Source: CAD feature listing. Evaluate the final solid. Frame: model axes, mm. A direction names the side the tool comes from. Give positions to 0.01 mm unless a question says otherwise; leave off trailing zeros. Loops run counter-clockwise (first coordinate to the right, second up) from the corner with the lowest first, then second, coordinate; pieces in that order, holes last. Notation, with made-up numbers: M 46.25,28 L 91.25,28 A26 cw 91.25,43 Z; hole C 47,10.5 d1. An arc over 180 degrees is marked long. Answer in a Markdown table with one row per item.
Autodesk Inventor part; units mm, degrees
ref_plane "YZ Plane" through (0, 0, 0) normal (1, 0, 0) x (0, 1, 0)
ref_plane "XZ Plane" through (0, 0, 0) normal (0, 1, 0) x (-1, 0, 0)
ref_plane "XY Plane" through (0, 0, 0) normal (0, 0, 1) x (1, 0, 0)
sketch "Sketch1" plane through (0, 0, 0) normal (0, 1, 0) x (-1, 0, 0)
  line L0 (0, 0) -> (19, 0) construction
  line L1 (19, -5) -> (19, -15.5)
  line L2 (19, 0) -> (16, 0) construction
  line L3 (16, 0) -> (16, -5)
  line L4 (16, -5) -> (19, -5)
  circle A0 centre (0, 0) radius 14.5
  line L5 (19, -15.5) -> (0, -15.5)
  line L6 (0, 0) -> (0, 19.3776) construction
  line L7 (19, 5) -> (19, 15.5)
  line L8 (16, 0) -> (16, 5)
  line L9 (16, 5) -> (19, 5)
  line L10 (19, 15.5) -> (0, 15.5)
  line L11 (0, 0) -> (0, -19.3776) construction
  line L12 (-19, -5) -> (-19, -15.5)
  line L13 (-16, 0) -> (-16, -5)
  line L14 (-16, -5) -> (-19, -5)
  line L15 (-19, -15.5) -> (0, -15.5)
  line L16 (-16, 0) -> (-16, 5)
  line L17 (-16, 5) -> (-19, 5)
  line L18 (-19, 5) -> (-19, 15.5)
  line L19 (-19, 15.5) -> (0, 15.5)
  dimension "d1" = 19
  dimension "d2" = 15.5
  dimension "d5" = 5
extrude "Extrusion1" add sketch "Sketch1" along normal blind 3 contours L1 L5 L15 L12 L14 L13 L16 L17 L18 L19 L10 L7 L9 L8 L3 L4 | A0
sketch "Sketch4" plane through (0, 3, 0) normal (0, 1, 0) x (1, 0, 0)
  circle A0 centre (0, 0) radius 15
  dimension "d14" = 30
extrude "Extrusion4" cut sketch "Sketch4" against normal up to surface (3 mm away)
sketch "Sketch5" plane through (0, 0, 0) normal (0, -1, 0) x (1, 0, 0)
  line L0 (19, -15.5) -> (-19, -15.5)
  line L1 (-19, -15.5) -> (-19, -16.5)
  line L2 (-19, -16.5) -> (19, -16.5)
  line L3 (19, -16.5) -> (19, -15.5)
  line L4 (-19, 15.5) -> (19, 15.5)
  line L5 (19, 15.5) -> (19, 16.5)
  line L6 (19, 16.5) -> (-19, 16.5)
  line L7 (-19, 16.5) -> (-19, 15.5)
  point P0 (0, 0)
  dimension "d17" = 1
  dimension "d18" = 1
extrude "Extrusion5" add sketch "Sketch5" against normal up to surface (3 mm away)
properties part number "SoporteSensor"
1) Section C-C, the plane y = 1.9. Return loops of the section in (x, z), then the cut area to 3 significant figures.
Reply:
| item | result |
|---|---|
| outline | M -19,-16.5 L 19,-16.5 L 19,-5 L 16,-5 L 16,5 L 19,5 L 19,16.5 L -19,16.5 L -19,5 L -16,5 L -16,-5 L -19,-5 Z; hole C 0,0 d30 |
| area | 487 mm² |
2) Set-up query: faces 4 (the flat face through (-17, 1, -5)), 5 (the flat face through (0, 1, 16.5)), 6 (the flat face through (17, 1, 5)). Return all of +Z, -Z, +X, -X, +Y, -Y with unobstructed straight access to the full face (end or side cutting, diameter ignored); none if empty.
Reply:
| item | result |
|---|---|
| face 4 | -X, +Y, -Y |
| face 5 | +Z, +X, -X, +Y, -Y |
| face 6 | +X, +Y, -Y |
3) Section B-B, the plane x = 0. Return loops of the section in (y, z).
Reply:
| item | result |
|---|---|
| outline | M 0,-16.5 L 3,-16.5 L 3,-15 L 0,-15 Z; M 0,15 L 3,15 L 3,16.5 L 0,16.5 Z |
4) Pin query (flat end, axial travel): pin 1 Ø1.5 at (y, z) = (2, 0.5) entering from +X. Return the tip coordinate at first contact, or that it passes through.
Reply:
| item | result |
|---|---|
| pin 1 | stops at x = 16 |
5) Material intervals for L1, parallel to Z at x = 16.5, y = 0.3; L2, parallel to Z at x = 0, y = 1.3; L3, parallel to X at y = 1.4, z = 0, sorted ascending.
Reply:
| item | result |
|---|---|
| L1 | z = -16.5 to -5, 5 to 16.5 |
| L2 | z = -16.5 to -15, 15 to 16.5 |
| L3 | x = -16 to -15, 15 to 16 |
6) Section A-A, the plane z = 0. Return loops of the section in (x, y).
Reply:
| item | result |
|---|---|
| outline | M -16,0 L -15,0 L -15,3 L -16,3 Z; M 15,0 L 16,0 L 16,3 L 15,3 Z |
7) Pull-direction query (X, two-part tool) for faces 1 (the cylindrical face through (-14.985, 1.521, -0.66)), 2 (the flat face through (-19, 1, 11)), 3 (the flat face through (16, 1, 0)); classes: released by +X, released by -X, zero draft, split by the parting line, or undercut.
Reply:
| item | result |
|---|---|
| face 1 | undercut |
| face 2 | released by -X |
| face 3 | released by +X |
